```python
from build123d import *

# Parameters (mm, degrees)
EXTRUDE_1_DEPTH     = 1.6
VIAHOLELAYER_R      = 1.6
CUT_EXTRUDE_2_DEPTH = 1.6


# Read off the part's stored shape, not the designer's step: 凸台-拉伸1
with BuildPart() as part:
    # 凸台-拉伸1 outline → 凸台-拉伸1 (new body)
    with BuildSketch(Plane.XY):
        with BuildLine():
            Line((28.205781396, 97.600023259), (28.205781396, 41.846499647))
            ThreePointArc((28.205781396, 41.846499647), (28.269280711, 41.783294645), (28.206371386, 41.719502388))
            ThreePointArc((28.206371386, 41.719502388), (29.251799434, 39.322351184), (31.68600117, 38.36636185))
            ThreePointArc((31.68600117, 38.36636185), (31.7485964, 38.431616297), (31.81297676, 38.3681224))
            Line((31.81297676, 38.3681224), (95.0595, 38.3681224))
            ThreePointArc((95.0595, 38.3681224), (95.123585364, 38.431619702), (95.186489208, 38.366951722))
            ThreePointArc((95.186489208, 38.366951722), (95.186493897, 38.366661387), (95.186497259, 38.366371034))
            ThreePointArc((95.186497259, 38.366371034), (97.583648579, 39.411799201), (98.539637791, 41.846001151))
            ThreePointArc((98.539637791, 41.846001151), (98.474383338, 41.908596378), (98.537877235, 41.972976741))
            Line((98.537877235, 41.972976741), (98.537877235, 97.726500353))
            ThreePointArc((98.537877235, 97.726500353), (98.474379933, 97.79058572), (98.539047919, 97.85348956))
            ThreePointArc((98.539047919, 97.85348956), (98.539338257, 97.85349425), (98.539628614, 97.853497612))
            ThreePointArc((98.539628614, 97.853497612), (97.494200566, 100.250648816), (95.05999883, 101.20663815))
            ThreePointArc((95.05999883, 101.20663815), (94.9974036, 101.141383703), (94.93302324, 101.2048776))
            Line((94.93302324, 101.2048776), (31.6865, 101.2048776))
            ThreePointArc((31.6865, 101.2048776), (31.622414636, 101.141380298), (31.559510792, 101.206048278))
            ThreePointArc((31.559510792, 101.206048278), (31.559506103, 101.206338613), (31.559502741, 101.206628966))
            ThreePointArc((31.559502741, 101.206628966), (29.162358971, 100.161208634), (28.206361808, 97.727020607))
            ThreePointArc((28.206361808, 97.727020607), (28.206656954, 97.727017223), (28.206952081, 97.727012467))
            ThreePointArc((28.206952081, 97.727012467), (28.271622765, 97.663523259), (28.206952081, 97.600034052))
            ThreePointArc((28.206952081, 97.600034052), (28.206366763, 97.600025958), (28.205781396, 97.600023259))
        make_face()
    extrude(amount=EXTRUDE_1_DEPTH)

    # ViaHoleLayer → 切除-拉伸2 (cut)
    with BuildSketch(Plane.XY):
        with Locations((95.12300254, 97.79)):
            Circle(VIAHOLELAYER_R)
        with Locations((95.12300254, 41.783)):
            Circle(VIAHOLELAYER_R)
        with Locations((31.623, 41.783)):
            Circle(VIAHOLELAYER_R)
        with Locations((31.623, 97.79)):
            Circle(VIAHOLELAYER_R)
    extrude(amount=CUT_EXTRUDE_2_DEPTH, mode=Mode.SUBTRACT)


solid = part.part
```
Model file for the job. Use its own axes, mm. Coordinates: 2 decimals unless noted, no trailing zeros. Use a Markdown table: item, result. Add a question column.
Item 1: Two-plate mould, pull along Y, no slides. Class faces 1 (the face through (32.483, 43.132, 0.789)), 2 (the face through (97.521, 100.224, 0.789)), 3 (the face through (93.525, 41.853, 0.789)), 4 (the face through (29.225, 39.349, 0.789)): pulls with the +Y half, pulls with the -Y half, needs draft (parallel to the pull), parting line crosses it, or undercut.
Item 2: Drill centre lines: line 1 along X through (y, z) = (97.79, 0.7); line 2 along Y through (x, z) = (85.5, 0.55); line 3 along X through (y, z) = (90, 0.15). Where is each one in solid material? Low to high.
Item 3: Drop flat-ended pins along their axis: pin 1 (1.9 mm diameter, centred on x = 95.12, y = 41.78, fed in from -Z); pin 2 (0.5 mm diameter, centred on x = 62.5, z = 0.5, fed in from -Y). Give the stop position or say it passes through.
A:
| question | item | result |
|---|---|---|
| 1 | face 1 | undercut |
| 1 | face 2 | pulls with the +Y half |
| 1 | face 3 | undercut |
| 1 | face 4 | pulls with the -Y half |
| 2 | line 1 | x = 28.21 to 30.02, 33.22 to 93.52, 96.72 to 98.47 |
| 2 | line 2 | y = 38.37 to 101.2 |
| 2 | line 3 | x = 28.21 to 98.54 |
| 3 | pin 1 | passes through |
| 3 | pin 2 | stops at y = 38.37 |
